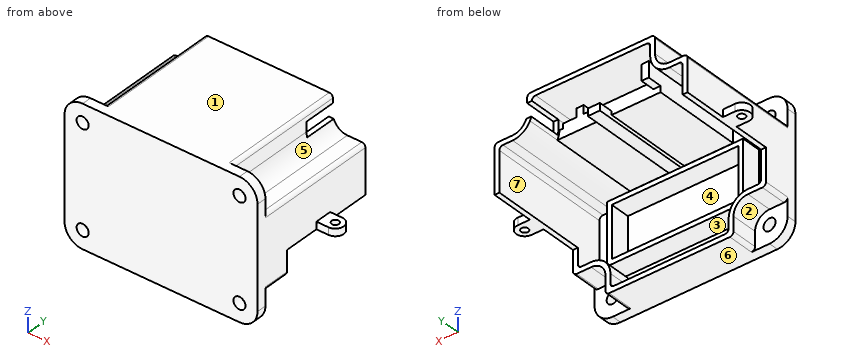
from build123d import *

# Parameters (mm, degrees)
EXTRUDE_1_DEPTH     = 4
SKETCH_1_3_R        = 2.5
CUT_EXTRUDE_1_DEPTH = 5
SKETCH_1_4_W        = 52.5
SKETCH_1_4_H        = 21.3
EXTRUDE_2_DEPTH     = 12.2
EXTRUDE_5_DEPTH     = 15
SKETCH_1_8_W        = 2
SKETCH_1_8_H        = 5
EXTRUDE_7_DEPTH     = 55
EXTRUDE_8_DEPTH     = 41
CUT_EXTRUDE_START   = -51.1
SKETCH_4_W          = 6
SKETCH_4_H          = 13.5
CUT_EXTRUDE_2_DEPTH = 2.5
SKETCH_7_W          = 37.5
SKETCH_7_H          = 3.5
CUT_EXTRUDE_3_DEPTH = 37
SKETCH_1_12_W       = 3
SKETCH_1_12_H       = 6.5
EXTRUDE_10_DEPTH    = 41
SKETCH_7_4_W        = 5
SKETCH_7_4_H        = 1.5
EXTRUDE_12_DEPTH    = 6
SKETCH_1_13_W       = 3
SKETCH_1_13_H       = 6.5
EXTRUDE_13_DEPTH    = 47
EXTRUDE_START       = 6
SKETCH_7_5_W        = 5
SKETCH_7_5_H        = 1.5
EXTRUDE_14_DEPTH    = 43
EXTRUDE_START_2     = -28.55
SKETCH_8_R          = 1.5
EXTRUDE_15_DEPTH    = 3
EXTRUDE_START_3     = -33.55
SKETCH_8_3_R        = 1.5
EXTRUDE_16_DEPTH    = 3


with BuildPart() as part:
    # Эскиз1 → Бобышка-Вытянуть1 (new body)
    with BuildSketch(Plane(origin=(0, 0, 0), x_dir=(1, 0, 0), z_dir=(0, 1, 0))):
        with BuildLine():
            Line((-65.1, 49.6), (0, 49.6))
            ThreePointArc((0, 49.6), (5.303300859, 47.403300859), (7.5, 42.1))
            Line((7.5, 42.1), (7.5, 0))
            ThreePointArc((7.5, 0), (5.303300859, -5.303300859), (0, -7.5))
            Line((0, -7.5), (-65.1, -7.5))
            ThreePointArc((-65.1, -7.5), (-70.403300859, -5.303300859), (-72.6, 0))
            Line((-72.6, 0), (-72.6, 42.1))
            ThreePointArc((-72.6, 42.1), (-70.403300859, 47.403300859), (-65.1, 49.6))
        make_face()
    extrude(amount=EXTRUDE_1_DEPTH)

    # Эскиз1<3> → Вырез-Вытянуть1 (cut)
    with BuildSketch(Plane(origin=(0, 0, 0), x_dir=(1, 0, 0), z_dir=(0, 1, 0))):
        with Locations(Location((-65.1, 42.1, 0), (0, 0, 270))):
            Circle(SKETCH_1_3_R)
        with Locations(Location((0, 42.1, 0), (0, 0, 90))):
            Circle(SKETCH_1_3_R)
        with Locations(Location((0, 0, 0), (0, 0, 270))):
            Circle(SKETCH_1_3_R)
        with Locations(Location((-65.1, 0, 0), (0, 0, 90))):
            Circle(SKETCH_1_3_R)
    extrude(amount=CUT_EXTRUDE_1_DEPTH, mode=Mode.SUBTRACT)

    # Эскиз1<4> → Бобышка-Вытянуть2 (add)
    with BuildSketch(Plane(origin=(0, 0, 0), x_dir=(1, 0, 0), z_dir=(0, 1, 0))):
        with BuildLine():
            ThreePointArc((-59.697222936, 36.2), (-60.230200598, 35.752949206), (-60.8, 35.35389001))
            Line((-60.8, 35.35389001), (-60.8, 10.9))
            Line((-60.8, 10.9), (-4.3, 10.9))
            Line((-4.3, 10.9), (-4.3, 35.35389001))
            ThreePointArc((-4.3, 35.35389001), (-4.869799402, 35.752949206), (-5.402777064, 36.2))
            Line((-5.402777064, 36.2), (-59.697222936, 36.2))
        make_face()
        with Locations((-32.55, 23.55)):
            Rectangle(SKETCH_1_4_W, SKETCH_1_4_H, mode=Mode.SUBTRACT)
    extrude(amount=EXTRUDE_2_DEPTH)

    # Эскиз1<7> → Бобышка-Вытянуть5 (add)
    with BuildSketch(Plane(origin=(0, 0, 0), x_dir=(1, 0, 0), z_dir=(0, 1, 0))):
        with BuildLine():
            Line((-7.5, 49.6), (-57.6, 49.6))
            ThreePointArc((-57.6, 49.6), (-58.660660172, 49.160660172), (-59.1, 48.1))
            Line((-59.1, 48.1), (-59.1, 42.1))
            ThreePointArc((-59.1, 42.1), (-60.857359313, 37.857359313), (-65.1, 36.1))
            Line((-65.1, 36.1), (-71.1, 36.1))
            ThreePointArc((-71.1, 36.1), (-72.160660172, 35.660660172), (-72.6, 34.6))
            Line((-72.6, 34.6), (-72.6, 7.5))
            ThreePointArc((-72.6, 7.5), (-72.160660172, 6.439339828), (-71.1, 6))
            Line((-71.1, 6), (-65.1, 6))
            ThreePointArc((-65.1, 6), (-60.857359313, 4.242640687), (-59.1, 0))
            Line((-59.1, 0), (-59.1, -6))
            ThreePointArc((-59.1, -6), (-58.660660172, -7.060660172), (-57.6, -7.5))
            Line((-57.6, -7.5), (-7.5, -7.5))
            ThreePointArc((-7.5, -7.5), (-6.439339828, -7.060660172), (-6, -6))
            Line((-6, -6), (-6, 0))
            ThreePointArc((-6, 0), (-4.242640687, 4.242640687), (0, 6))
            Line((0, 6), (6, 6))
            ThreePointArc((6, 6), (7.060660172, 6.439339828), (7.5, 7.5))
            Line((7.5, 7.5), (7.5, 21.05))
            Line((7.5, 21.05), (5.5, 21.05))
            Line((5.5, 21.05), (5.5, 9.5))
            ThreePointArc((5.5, 9.5), (5.060660172, 8.439339828), (4, 8))
            Line((4, 8), (0, 8))
            ThreePointArc((0, 8), (-5.656854249, 5.656854249), (-8, 0))
            Line((-8, 0), (-8, -4))
            ThreePointArc((-8, -4), (-8.439339828, -5.060660172), (-9.5, -5.5))
            Line((-9.5, -5.5), (-55.6, -5.5))
            ThreePointArc((-55.6, -5.5), (-56.660660172, -5.060660172), (-57.1, -4))
            Line((-57.1, -4), (-57.1, 0))
            ThreePointArc((-57.1, 0), (-59.443145751, 5.656854249), (-65.1, 8))
            Line((-65.1, 8), (-69.1, 8))
            ThreePointArc((-69.1, 8), (-70.160660172, 8.439339828), (-70.6, 9.5))
            Line((-70.6, 9.5), (-70.6, 32.6))
            ThreePointArc((-70.6, 32.6), (-70.160660172, 33.660660172), (-69.1, 34.1))
            Line((-69.1, 34.1), (-65.1, 34.1))
            ThreePointArc((-65.1, 34.1), (-59.443145751, 36.443145751), (-57.1, 42.1))
            Line((-57.1, 42.1), (-57.1, 46.1))
            ThreePointArc((-57.1, 46.1), (-56.660660172, 47.160660172), (-55.6, 47.6))
            Line((-55.6, 47.6), (-9.5, 47.6))
            ThreePointArc((-9.5, 47.6), (-8.439339828, 47.160660172), (-8, 46.1))
            Line((-8, 46.1), (-8, 42.1))
            ThreePointArc((-8, 42.1), (-5.656854249, 36.443145751), (0, 34.1))
            Line((0, 34.1), (4, 34.1))
            ThreePointArc((4, 34.1), (5.060660172, 33.660660172), (5.5, 32.6))
            Line((5.5, 32.6), (5.5, 26.05))
            Line((5.5, 26.05), (7.5, 26.05))
            Line((7.5, 26.05), (7.5, 34.6))
            ThreePointArc((7.5, 34.6), (7.060660172, 35.660660172), (6, 36.1))
            Line((6, 36.1), (0, 36.1))
            ThreePointArc((0, 36.1), (-4.242640687, 37.857359313), (-6, 42.1))
            Line((-6, 42.1), (-6, 48.1))
            ThreePointArc((-6, 48.1), (-6.439339828, 49.160660172), (-7.5, 49.6))
        make_face()
    extrude(amount=EXTRUDE_5_DEPTH)

    # Эскиз1<8> → Бобышка-Вытянуть7 (add)
    with BuildSketch(Plane(origin=(0, 0, 0), x_dir=(1, 0, 0), z_dir=(0, 1, 0))):
        with BuildLine():
            Line((-70.6, 21.05), (-72.6, 21.05))
            Line((-72.6, 21.05), (-72.6, 7.5))
            ThreePointArc((-72.6, 7.5), (-72.160660172, 6.439339828), (-71.1, 6))
            Line((-71.1, 6), (-65.1, 6))
            ThreePointArc((-65.1, 6), (-60.857359313, 4.242640687), (-59.1, 0))
            Line((-59.1, 0), (-59.1, -6))
            ThreePointArc((-59.1, -6), (-58.660660172, -7.060660172), (-57.6, -7.5))
            Line((-57.6, -7.5), (-7.5, -7.5))
            ThreePointArc((-7.5, -7.5), (-6.439339828, -7.060660172), (-6, -6))
            Line((-6, -6), (-6, 0))
            ThreePointArc((-6, 0), (-4.242640687, 4.242640687), (0, 6))
            Line((0, 6), (6, 6))
            ThreePointArc((6, 6), (7.060660172, 6.439339828), (7.5, 7.5))
            Line((7.5, 7.5), (7.5, 21.05))
            Line((7.5, 21.05), (5.5, 21.05))
            Line((5.5, 21.05), (5.5, 9.5))
            ThreePointArc((5.5, 9.5), (5.060660172, 8.439339828), (4, 8))
            Line((4, 8), (0, 8))
            ThreePointArc((0, 8), (-4.242640687, 6.782329983), (-7.193747285, 3.5))
            ThreePointArc((-7.193747285, 3.5), (-7.795831523, 1.795831523), (-8, 0))
            Line((-8, 0), (-8, -4))
            ThreePointArc((-8, -4), (-8.439339828, -5.060660172), (-9.5, -5.5))
            Line((-9.5, -5.5), (-15.1, -5.5))
            Line((-15.1, -5.5), (-18.1, -5.5))
            Line((-18.1, -5.5), (-47, -5.5))
            Line((-47, -5.5), (-50, -5.5))
            Line((-50, -5.5), (-55.6, -5.5))
            ThreePointArc((-55.6, -5.5), (-56.660660172, -5.060660172), (-57.1, -4))
            Line((-57.1, -4), (-57.1, 0))
            ThreePointArc((-57.1, 0), (-57.304168477, 1.795831523), (-57.906252715, 3.5))
            ThreePointArc((-57.906252715, 3.5), (-60.857359313, 6.782329983), (-65.1, 8))
            Line((-65.1, 8), (-69.1, 8))
            ThreePointArc((-69.1, 8), (-70.160660172, 8.439339828), (-70.6, 9.5))
            Line((-70.6, 9.5), (-70.6, 21.05))
        make_face()
        with Locations((6.5, 23.55)):
            Rectangle(SKETCH_1_8_W, SKETCH_1_8_H)
    extrude(amount=EXTRUDE_7_DEPTH)

    # Эскиз1<9> → Бобышка-Вытянуть8 (add)
    with BuildSketch(Plane(origin=(0, 0, 0), x_dir=(1, 0, 0), z_dir=(0, 1, 0))):
        with BuildLine():
            Line((-50, 3.5), (-50, 1))
            Line((-50, 1), (-47, 1))
            Line((-47, 1), (-47, -5.5))
            Line((-47, -5.5), (-18.1, -5.5))
            Line((-18.1, -5.5), (-18.1, 1))
            Line((-18.1, 1), (-15.1, 1))
            Line((-15.1, 1), (-15.1, -5.5))
            Line((-15.1, -5.5), (-9.5, -5.5))
            Line((-9.5, -5.5), (-9.5, 0))
            Line((-9.5, 0), (-8, 0))
            ThreePointArc((-8, 0), (-7.795831523, 1.795831523), (-7.193747285, 3.5))
            Line((-7.193747285, 3.5), (-50, 3.5))
        make_face()
    extrude(amount=EXTRUDE_8_DEPTH)

    # Эскиз4 → Вырез-Вытянуть2 (cut, symmetric)
    with BuildSketch(Plane.ZY.offset(59.1).offset(CUT_EXTRUDE_START)):
        with Locations((1, 48.25)):
            Rectangle(SKETCH_4_W, SKETCH_4_H)
    extrude(amount=CUT_EXTRUDE_2_DEPTH, both=True, mode=Mode.SUBTRACT)

    # Эскиз7 → Вырез-Вытянуть3 (cut)
    with BuildSketch(Plane(origin=(0, 41, 0), x_dir=(1, 0, 0), z_dir=(0, 1, 0))):
        with Locations((-28.25, -3.75)):
            Rectangle(SKETCH_7_W, SKETCH_7_H)
    extrude(amount=-CUT_EXTRUDE_3_DEPTH, mode=Mode.SUBTRACT)

    # Эскиз1<12> → Бобышка-Вытянуть10 (add)
    with BuildSketch(Plane(origin=(0, 0, 0), x_dir=(1, 0, 0), z_dir=(0, 1, 0))):
        with Locations((-16.6, -2.25)):
            Rectangle(SKETCH_1_12_W, SKETCH_1_12_H)
    extrude(amount=EXTRUDE_10_DEPTH)

    # Эскиз7<4> → Бобышка-Вытянуть12 (add)
    with BuildSketch(Plane(origin=(0, 41, 0), x_dir=(1, 0, 0), z_dir=(0, 1, 0))):
        with Locations((-27.2, 2.75)):
            Rectangle(SKETCH_7_4_W, SKETCH_7_4_H)
    extrude(amount=EXTRUDE_12_DEPTH)

    # Эскиз1<13> → Бобышка-Вытянуть13 (add)
    with BuildSketch(Plane(origin=(0, 0, 0), x_dir=(1, 0, 0), z_dir=(0, 1, 0))):
        with Locations((-48.5, -2.25)):
            Rectangle(SKETCH_1_13_W, SKETCH_1_13_H)
    extrude(amount=EXTRUDE_13_DEPTH)

    # Эскиз7<5> → Бобышка-Вытянуть14 (add)
    with BuildSketch(Plane(origin=(0, 41, 0), x_dir=(1, 0, 0), z_dir=(0, 1, 0)).offset(EXTRUDE_START)):
        with Locations((-27.2, 4.25)):
            Rectangle(SKETCH_7_5_W, SKETCH_7_5_H)
    extrude(amount=-EXTRUDE_14_DEPTH)

    # Эскиз8 → Бобышка-Вытянуть15 (add)
    with BuildSketch(Plane.XY.offset(7.5).offset(EXTRUDE_START_2)):
        with BuildLine():
            Line((-72.6, 37), (-77.6, 37))
            ThreePointArc((-77.6, 37), (-81.1, 33.5), (-77.6, 30))
            Line((-77.6, 30), (-72.6, 30))
            Line((-72.6, 30), (-72.6, 37))
        make_face()
        with Locations(Location((-77.6, 33.5, 0), (0, 0, 180))):
            Circle(SKETCH_8_R, mode=Mode.SUBTRACT)
    extrude(amount=EXTRUDE_15_DEPTH)

    # Эскиз8<3> → Бобышка-Вытянуть16 (add)
    with BuildSketch(Plane.XY.offset(7.5).offset(EXTRUDE_START_3)):
        with BuildLine():
            ThreePointArc((12.5, 37), (16, 33.5), (12.5, 30))
            Line((12.5, 30), (7.5, 30))
            Line((7.5, 30), (7.5, 37))
            Line((7.5, 37), (12.5, 37))
        make_face()
        with Locations((12.5, 33.5)):
            Circle(SKETCH_8_3_R, mode=Mode.SUBTRACT)
    extrude(amount=EXTRUDE_16_DEPTH)


solid = part.part
For this review, take the finished solid that the model builds, in its own axes (mm). Face numbers are marked on the shaded views. A direction names the side the tool comes from. Round coordinates to 2 decimals unless told otherwise and drop trailing zeros. Order: outer loops, then holes, each group sorted by start corner. A loop starts at its lowest first (then second) coordinate and runs counter-clockwise, first axis right, second up. Notation, with made-up numbers: M 43,27.25 L 79,27.25 A26 cw 79,45.25 Z; hole C 19,-7 d10. An arc over 180 degrees is marked long. Write each question's results on one line, items separated by ' | '. Start each with the question number.
1. Add section C-C (y = 25). State how many separate pieces and enclosed holes the cut face has, then the cut area to 3 significant figures.
2. Tool access review of the marked faces 1, 2 and 3: name each direction out of +Z, -Z, +X, -X, +Y, -Y from which nothing blocks a thin tool from reaching the whole face with its end or side.
3. To check wall thickness, follow L1, parallel to Z at x = -65.1, y = 3.05; L2, parallel to X at y = 1, z = -42; L3, parallel to Z at x = -37, y = 13.5. State the ranges of each line that lie inside material, in increasing order. Write a range as [from, to].
4. Add section B-B (x = -43). State the section outline as (y, z) points.
5. Add section A-A (z = -15). State the section outline as (x, y) points.
6. Draft analysis for pull direction X (two halves, no side actions). For the marked faces 4, 5, 6 and 7, state which applies: pulls with the +X half, pulls with the -X half, needs draft (parallel to the pull), parting line crosses it, or undercut.
7. Clearance check with flat-ended pins moving along their axes: pin 1 Ø3 at (y, z) = (11.5, -44.5) entering from +X; pin 2 Ø0.9 at (x, z) = (-74.5, -19) entering from -Y; pin 3 Ø5 at (y, z) = (24.5, 1) entering from +X; pin 4 Ø3 at (y, z) = (47.5, -28.5) entering from -X. State where each tip first meets the part, or that it passes through.
Output values:
1) separate pieces: 1 | enclosed holes: 2 | area: 522 mm^2
2) face 1: +Z, +X, -X, +Y, -Y | face 2: -Z, -X, +Y | face 3: +Y
3) L1: [-49.6, -44.6], [-39.6, -2.5], [2.5, 7.5] | L2: [-72.6, -67.6], [-62.6, -2.5], [2.5, 7.5] | L3: [-49.6, -47.6], [-3.5, 2], [5.5, 7.5]
4) outline: M 0,-49.6 L 15,-49.6 L 15,-47.6 L 4,-47.6 L 4,-36.2 L 12.2,-36.2 L 12.2,-34.2 L 4,-34.2 L 4,-12.9 L 12.2,-12.9 L 12.2,-10.9 L 4,-10.9 L 4,-3.5 L 41,-3.5 L 41,2 L 4,2 L 4,5.5 L 55,5.5 L 55,7.5 L 0,7.5 Z
5) outline: M -72.6,0 L 7.5,0 L 7.5,55 L 5.5,55 L 5.5,4 L -4.3,4 L -4.3,12.2 L -6.3,12.2 L -6.3,4 L -58.8,4 L -58.8,12.2 L -60.8,12.2 L -60.8,4 L -70.6,4 L -70.6,55 L -72.6,55 Z
6) face 4: undercut | face 5: pulls with the +X half | face 6: needs draft | face 7: undercut
7) pin 1: x = -6 | pin 2: y = 30 | pin 3: x = -5.81 | pin 4: through
